from build123d import *

# Parameters (mm, degrees)
MAIN_BASE_DIM_W                            = 76.2
MAIN_BASE_DIM_H                            = 50.8
MAIN_BASE_DEPTH                            = 2.54
LINKAGE_HOLDER_DIM_W                       = 38.1
LINKAGE_HOLDER_DIM_H                       = 19.05
LINKAGE_HOLDER_DEPTH                       = 50.8
LINKAGE_SLOT_DIM_W                         = 25.6
LINKAGE_SLOT_DIM_H                         = 1.4
LINKAGE_SLOT_DEPTH                         = 50.8
F_75IN_FILLET_R                            = 19.05
BOLT_HOLE_REACH                            = 101.355
BOLT_HOLE_DIM_R                            = 2.1828
BOLT_HEAD_DIM_R                            = 4.445
BOLT_HEAD_DEPTH                            = 5.5372
NUT_SLOT_DEPTH                             = 5.5372
CSK_FOR_10_FLAT_HEAD_MACHINE_SCREW_2_COUNT = 2
CSK_FOR_10_FLAT_HEAD_MACHINE_SCREW_2_PITCH = 33.488349187
CSK_FOR_10_FLAT_HEAD_MACHINE_SCREW_3_COUNT = 2
CSK_FOR_10_FLAT_HEAD_MACHINE_SCREW_3_PITCH = 57.15
CSK_FOR_10_FLAT_HEAD_MACHINE_SCREW_4_COUNT = 2
CSK_FOR_10_FLAT_HEAD_MACHINE_SCREW_4_PITCH = 33.488349187
CORNER_CUT_DEPTH                           = 2.54
F_1IN_FILLET_R                             = 2.54


with BuildPart() as part:
    # Main_Base_Dim → Main_Base (new body)
    with BuildSketch(Plane(origin=(0, 0, 0), x_dir=(1, 0, 0), z_dir=(0, 1, 0))):
        with Locations((38.1, 25.4)):
            Rectangle(MAIN_BASE_DIM_W, MAIN_BASE_DIM_H)
    extrude(amount=MAIN_BASE_DEPTH)

    # Linkage_Holder_Dim → Linkage_Holder (add)
    with BuildSketch(Plane(origin=(0, 2.54, 0), x_dir=(1, 0, 0), z_dir=(0, 1, 0))):
        with Locations((38.1, 25.4)):
            Rectangle(LINKAGE_HOLDER_DIM_W, LINKAGE_HOLDER_DIM_H)
    extrude(amount=LINKAGE_HOLDER_DEPTH)

    # Linkage_Slot_Dim → Linkage_Slot (cut)
    with BuildSketch(Plane(origin=(0, 53.34, 0), x_dir=(1, 0, 0), z_dir=(0, 1, 0))):
        with Locations((38.1, 25.4)):
            Rectangle(LINKAGE_SLOT_DIM_W, LINKAGE_SLOT_DIM_H)
    extrude(amount=-LINKAGE_SLOT_DEPTH, mode=Mode.SUBTRACT)

    # .75in_Fillet
    # the kernel refuses this fillet: 19.05 mm, written as the material it takes off along each edge
    with BuildSketch(Plane(origin=(57.15, 53.34, -82.55), x_dir=(0, -1, 0), z_dir=(0, 0, 1)), Plane(origin=(19.05, 53.34, 31.75), x_dir=(0, -1, 0), z_dir=(0, 0, -1))) as f_75in_fillet_piece_1:
        with BuildLine():
            CenterArc((F_75IN_FILLET_R, -F_75IN_FILLET_R), F_75IN_FILLET_R, 90, 90)
            Line((0, -F_75IN_FILLET_R), (0, 0))
            Line((0, 0), (F_75IN_FILLET_R, 0))
        make_face()
    extrude(amount=114.3, mode=Mode.SUBTRACT)

    # Bolt_Hole: up to this face of the body (flat: up to its plane)
    bolt_hole_end = Plane(part.part.faces().sort_by_distance((38.1, 26.089428348, -34.925))[0])
    # Bolt_Hole_Dim → Bolt_Hole (cut, up to the picked face)
    with BuildSketch(Plane.XY.offset(-15.875), mode=Mode.PRIVATE) as bolt_hole_sk1:
        with Locations((38.1, 34.29)):
            Circle(BOLT_HOLE_DIM_R)
    bolt_hole_tool1 = split(extrude(bolt_hole_sk1.sketch, amount=-BOLT_HOLE_REACH, mode=Mode.PRIVATE), bisect_by=bolt_hole_end, keep=Keep.BOTH, mode=Mode.PRIVATE)
    add(bolt_hole_tool1.solids().sort_by(Axis((38.1, 34.29, -15.875), (0, 0, -1)))[0], mode=Mode.SUBTRACT)

    # Bolt_Head_Dim → Bolt_Head (cut)
    with BuildSketch(Plane.XY.offset(-15.875)):
        with Locations((38.1, 34.29)):
            Circle(BOLT_HEAD_DIM_R)
    extrude(amount=-BOLT_HEAD_DEPTH, mode=Mode.SUBTRACT)

    # Nut_Slot_Dim → Nut_Slot (cut)
    with BuildSketch(Plane(origin=(0, 0, -34.925), x_dir=(-1, 0, 0), z_dir=(0, 0, -1))):
        Polygon((-35.6235, 38.579423825), (-40.5765, 38.579423825), (-43.053, 34.29), (-40.5765, 30.000576175), (-35.6235, 30.000576175), (-33.147, 34.29), align=None)
    extrude(amount=-NUT_SLOT_DEPTH, mode=Mode.SUBTRACT)

    # Sketch9 → CSK for #10 Flat Head Machine Screw (100)1 (revolve, cut)
    with BuildSketch(Plane(origin=(9.525, 2.54, -25.4), x_dir=(0, 0, 1), z_dir=(1, 0, 0))):
        Polygon((0, 0), (0, 2.54), (2.5527, 2.54), (2.5527, 1.960808018), (4.8895, 0), align=None)
    csk_for_10_flat_head_machine_screw_100 = revolve(axis=Axis((9.525, 8.89, -25.4), (0, -1, 0)), mode=Mode.SUBTRACT)

    # CSK for _10 Flat Head Machine Screw  2: CSK for #10 Flat Head Machine Screw (100)1 ×2
    with Locations(*[Vector(0.8532818336519591, 0, -0.5214500094539748) * (i * CSK_FOR_10_FLAT_HEAD_MACHINE_SCREW_2_PITCH) for i in range(1, CSK_FOR_10_FLAT_HEAD_MACHINE_SCREW_2_COUNT)]):
        add(csk_for_10_flat_head_machine_screw_100, mode=Mode.SUBTRACT)

    # CSK for _10 Flat Head Machine Screw  3: CSK for #10 Flat Head Machine Screw (100)1 ×2
    with Locations(*[(i * CSK_FOR_10_FLAT_HEAD_MACHINE_SCREW_3_PITCH, 0, 0) for i in range(1, CSK_FOR_10_FLAT_HEAD_MACHINE_SCREW_3_COUNT)]):
        add(csk_for_10_flat_head_machine_screw_100, mode=Mode.SUBTRACT)

    # CSK for _10 Flat Head Machine Screw  4: CSK for #10 Flat Head Machine Screw (100)1 ×2
    with Locations(*[Vector(0.853281833651959, 0, 0.521450009453975) * (i * CSK_FOR_10_FLAT_HEAD_MACHINE_SCREW_4_PITCH) for i in range(1, CSK_FOR_10_FLAT_HEAD_MACHINE_SCREW_4_COUNT)]):
        add(csk_for_10_flat_head_machine_screw_100, mode=Mode.SUBTRACT)

    # Screw_Hole cone 1 section (through the dimple's axis) → Screw_Hole (revolve, cut)
    with BuildSketch(Plane(origin=(9.525, 2.54, -25.4), x_dir=(0, 0, 1), z_dir=(1, 0, 0))):
        Polygon((0, 0), (4.6, 0), (0, 4.6), align=None)
    revolve(axis=Axis((9.525, 2.54, -25.4), (0, -1, 0)), mode=Mode.SUBTRACT)

    # Screw_Hole cone 2 section (through the dimple's axis) → Screw_Hole cone 2 (revolve, cut)
    with BuildSketch(Plane(origin=(38.1, 2.54, -42.8625), x_dir=(0, 0, 1), z_dir=(1, 0, 0))):
        Polygon((0, 0), (4.6, 0), (0, 4.6), align=None)
    revolve(axis=Axis((38.1, 2.54, -42.8625), (0, -1, 0)), mode=Mode.SUBTRACT)

    # Screw_Hole cone 3 section (through the dimple's axis) → Screw_Hole cone 3 (revolve, cut)
    with BuildSketch(Plane(origin=(66.675, 2.54, -25.4), x_dir=(0, 0, 1), z_dir=(1, 0, 0))):
        Polygon((0, 0), (4.6, 0), (0, 4.6), align=None)
    revolve(axis=Axis((66.675, 2.54, -25.4), (0, -1, 0)), mode=Mode.SUBTRACT)

    # Screw_Hole cone 4 section (through the dimple's axis) → Screw_Hole cone 4 (revolve, cut)
    with BuildSketch(Plane(origin=(38.1, 2.54, -7.9375), x_dir=(0, 0, 1), z_dir=(1, 0, 0))):
        Polygon((0, 0), (4.6, 0), (0, 4.6), align=None)
    revolve(axis=Axis((38.1, 2.54, -7.9375), (0, -1, 0)), mode=Mode.SUBTRACT)

    # Corner_Cut_Dim → Corner_Cut (cut)
    with BuildSketch(Plane(origin=(0, 2.54, 0), x_dir=(1, 0, 0), z_dir=(0, 1, 0))):
        Polygon((0, 0), (0, 19.05), (19.05, 0), align=None)
        Polygon((76.2, 0), (76.2, 19.05), (57.15, 0), align=None)
        Polygon((76.2, 50.8), (76.2, 31.75), (57.15, 50.8), align=None)
        Polygon((0, 31.75), (19.05, 50.8), (0, 50.8), align=None)
    extrude(amount=-CORNER_CUT_DEPTH, mode=Mode.SUBTRACT)

    # .1in_Fillet
    f_1in_fillet_edges = [part.edges().sort_by_distance(p)[0] for p in [
        (19.05, 2.54, -25.4),
        (19.05, 1.27, -50.8),
        (0, 1.27, -31.75),
        (38.1, 2.54, -15.875),
        (76.2, 1.27, -31.75),
        (57.15, 1.27, -50.8),
        (57.15, 2.54, -25.4),
        (76.2, 1.27, -19.05),
        (57.15, 1.27, 0),
        (38.1, 2.54, -34.925),
        (0, 1.27, -19.05),
        (19.05, 1.27, 0),
        (19.05, 18.415, -34.925),
        (57.15, 18.415, -34.925),
        (38.1, 53.34, -34.925),
        (38.1, 53.34, -34.925),
        (57.15, 18.415, -15.875),
        (19.05, 18.415, -15.875),
        (38.1, 53.34, -15.875),
        (38.1, 53.34, -15.875),
    ]]
    fillet(f_1in_fillet_edges, radius=F_1IN_FILLET_R)


solid = part.part
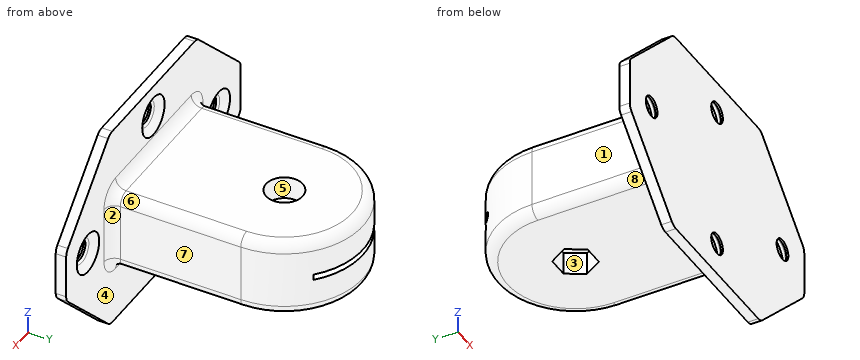
Input: part model. Units: mm. Frame: model coordinates. Face numbers are marked on the shaded views. A direction names the side the tool comes from. Give positions to 0.01 mm unless a question says otherwise; leave off trailing zeros. Loops run counter-clockwise (first coordinate to the right, second up) from the corner with the lowest first, then second, coordinate; pieces in that order, holes last. Notation, with made-up numbers: M 39.5,20.5 L 47.5,20.5 A14 cw 47.5,42.5 Z; hole C 65.25,-9 d2. An arc over 180 degrees is marked long. Use CSV: the item, a comma, the result in double quotes.
(1) Set-up query: the marked faces 4, 5, 6, 7 and 8. Return all of +Z, -Z, +X, -X, +Y, -Y with unobstructed straight access to the full face (end or side cutting, diameter ignored); none if empty.
Outcome:
face 4,"+Y"
face 5,"+Z"
face 6,"+Z, +X, +Y"
face 7,"+Z, -Z, +X, +Y"
face 8,"-Z, -X, +Y"
(2) Material intervals for L1, parallel to X at y = 0.1, z = -25.4; L2, parallel to Y at x = 38, z = -22; L3, parallel to X at y = 21, z = -30, sorted ascending. Write a range as [from, to].
Outcome:
L1,"x = [0, 6.97], [12.08, 64.12], [69.23, 76.2]"
L2,"y = [0, 32.11], [36.47, 53.34]"
L3,"x = [19.05, 57.15]"
(3) Pull-direction query (X, two-part tool) for the marked faces 1, 2 and 3; classes: pulls with the +X half, pulls with the -X half, needs draft (parallel to the pull), parting line crosses it, or undercut.
Outcome:
face 1,"pulls with the -X half"
face 2,"pulls with the +X half"
face 3,"undercut"
(4) Section B-B, the plane x = 38.1. Count the separate pieces of the cut face and the enclosed holes in it, plus the area to 3 significant figures.
Outcome:
separate pieces,"5"
enclosed holes,"0"
area,"865 mm²"
(5) Pin query (flat end, axial travel): P1, Ø2.5, axis at x = 38.5, y = 34, coming from the +Z side; P2, Ø20.5, axis at x = 42.5, y = 40, coming from the +Z side (3 decimals); P3, Ø5, axis at y = 7.5, z = -22.5, coming from the -X side; P4, Ø10, axis at x = 60.5, z = -41, coming from the +Y side. Return the tip coordinate at first contact, or that it passes through.
Outcome:
P1,"passes through"
P2,"stops at z = -15.875"
P3,"stops at x = 19.05"
P4,"stops at y = 2.54"
(6) Section A-A, the plane y = 13. Return loops of the section in (x, z) (3 decimals).
Outcome:
outline,"M 19.05,-32.385 A2.54 ccw 21.59,-34.925 L 54.61,-34.925 A2.54 ccw 57.15,-32.385 L 57.15,-18.415 A2.54 ccw 54.61,-15.875 L 21.59,-15.875 A2.54 ccw 19.05,-18.415 Z; hole M 25.3,-26.1 L 50.9,-26.1 L 50.9,-24.7 L 25.3,-24.7 Z"
